```python
from build123d import *

# Parameters (mm, degrees)
EXTRUDE_1_OUTLINE_R   = 35
EXTRUDE_1_OUTLINE_R_2 = 1.55
EXTRUDE_1_OUTLINE_R_3 = 30.05
EXTRUDE_1_DEPTH       = 10
SKETCH_2_R            = 33.525
SKETCH_2_R_2          = 18.525
EXTRUDE_1_2_DEPTH     = 4
SKETCH_3_R            = 1.55
CUT_EXTRUDE_1_DEPTH   = 51.497524692
CUT_EXTRUDE_2_DEPTH   = 6
SKETCH_8_R            = 35
SKETCH_8_R_2          = 30.05
CUT_EXTRUDE_3_DEPTH   = 2
SKETCH_9_R            = 3
CUT_EXTRUDE_4_DEPTH   = 2
SKETCH_10_R           = 1.55
CUT_EXTRUDE_5_DEPTH   = 51.139804547
SKETCH_11_R           = 3
CUT_EXTRUDE_6_DEPTH   = 2


# Read off the part's stored shape, not the designer's step: 凸台-拉伸1
with BuildPart() as part:
    # Extrude 1 outline → Extrude 1 (new body)
    with BuildSketch(Plane.XY):
        Circle(EXTRUDE_1_OUTLINE_R)
        with Locations((0, -32.5)):
            Circle(EXTRUDE_1_OUTLINE_R_2, mode=Mode.SUBTRACT)
        with Locations((-32.5, 0)):
            Circle(EXTRUDE_1_OUTLINE_R_2, mode=Mode.SUBTRACT)
        Circle(EXTRUDE_1_OUTLINE_R_3, mode=Mode.SUBTRACT)
        with Locations((32.5, 0)):
            Circle(EXTRUDE_1_OUTLINE_R_2, mode=Mode.SUBTRACT)
        with Locations((0, 32.5)):
            Circle(EXTRUDE_1_OUTLINE_R_2, mode=Mode.SUBTRACT)
    extrude(amount=EXTRUDE_1_DEPTH)

    # 草图2 → Extrude 1 2 (add)
    with BuildSketch(Plane.XY.offset(10)):
        Circle(SKETCH_2_R)
        Circle(SKETCH_2_R_2, mode=Mode.SUBTRACT)
    extrude(amount=-EXTRUDE_1_2_DEPTH)

    # 草图3 → 切除-拉伸1 (cut, through all)
    with BuildSketch(Plane(origin=(0, 0, 0), x_dir=(-1, 0, 0), z_dir=(0, 0, -1))):
        with Locations(Location((32.5, 0, 0), (0, 0, 180))):
            Circle(SKETCH_3_R)
        with Locations(Location((0, -32.5, 0), (0, 0, 180))):
            Circle(SKETCH_3_R)
        with Locations(Location((-32.5, 0, 0), (0, 0, 180))):
            Circle(SKETCH_3_R)
        with Locations(Location((0, 32.5, 0), (0, 0, 180))):
            Circle(SKETCH_3_R)
    extrude(amount=-CUT_EXTRUDE_1_DEPTH, mode=Mode.SUBTRACT)

    # 草图7 → 切除-拉伸2 (cut)
    with BuildSketch(Plane(origin=(0, 0, 0), x_dir=(-1, 0, 0), z_dir=(0, 0, -1))):
        with BuildLine():
            Line((15.025, 26.024063384), (17.5, 30.310889132))
            ThreePointArc((17.5, 30.310889132), (24.748737342, 24.748737342), (30.310889132, 17.5))
            Line((30.310889132, 17.5), (26.024063384, 15.025))
            ThreePointArc((26.024063384, 15.025), (21.248558775, 21.248558775), (15.025, 26.024063384))
        make_face()
    extrude(amount=-CUT_EXTRUDE_2_DEPTH, mode=Mode.SUBTRACT)

    # 草图8 → 切除-拉伸3 (cut)
    with BuildSketch(Plane(origin=(0, 0, 0), x_dir=(-1, 0, 0), z_dir=(0, 0, -1))):
        with Locations(Location((0, 0, 0), (0, 0, 30))):
            Circle(SKETCH_8_R)
        Circle(SKETCH_8_R_2, mode=Mode.SUBTRACT)
    extrude(amount=-CUT_EXTRUDE_3_DEPTH, mode=Mode.SUBTRACT)

    # 草图9 → 切除-拉伸4 (cut)
    with BuildSketch(Plane.XY.offset(10)):
        with Locations((0, 32.5)):
            Circle(SKETCH_9_R)
        with Locations((32.5, 0)):
            Circle(SKETCH_9_R)
        with Locations((0, -32.5)):
            Circle(SKETCH_9_R)
        with Locations((-32.5, 0)):
            Circle(SKETCH_9_R)
    extrude(amount=-CUT_EXTRUDE_4_DEPTH, mode=Mode.SUBTRACT)

    # 草图10 → 切除-拉伸5 (cut, through all)
    with BuildSketch(Plane.XY.offset(10)):
        with Locations((22.980970389, 22.980970389)):
            Circle(SKETCH_10_R)
        with Locations((22.980970389, -22.980970389)):
            Circle(SKETCH_10_R)
        with Locations((-22.980970389, -22.980970389)):
            Circle(SKETCH_10_R)
        with Locations((-22.980970389, 22.980970389)):
            Circle(SKETCH_10_R)
    extrude(amount=-CUT_EXTRUDE_5_DEPTH, mode=Mode.SUBTRACT)

    # 草图11 → 切除-拉伸6 (cut)
    with BuildSketch(Plane.XY.offset(10)):
        with Locations((22.980970389, 22.980970389)):
            Circle(SKETCH_11_R)
        with Locations((22.980970389, -22.980970389)):
            Circle(SKETCH_11_R)
        with Locations((-22.980970389, -22.980970389)):
            Circle(SKETCH_11_R)
        with Locations((-22.980970389, 22.980970389)):
            Circle(SKETCH_11_R)
    extrude(amount=-CUT_EXTRUDE_6_DEPTH, mode=Mode.SUBTRACT)


solid = part.part
```
Design review of the part built by this model. Coordinates are the model's own, in mm. A direction names the side the tool comes from. Round coordinates to 2 decimals unless told otherwise and drop trailing zeros. Order: outer loops, then holes, each group sorted by start corner. A loop starts at its lowest first (then second) coordinate and runs counter-clockwise, first axis right, second up. Notation, with made-up numbers: M 27,28 L 63,28 A13 cw 63,46 Z; hole C 60.5,56.25 d1. An arc over 180 degrees is marked long. Put each result on its own line as item: value.
Q1. To check wall thickness, follow line 1 (X direction, y = 0, z = 3.25); line 2 (Y direction, x = 23, z = 4.5); line 3 (Y direction, x = 0, z = 8.5) (3 decimals). State the ranges of each line that lie inside material, in increasing order.
Reported:
line 1: -35 to -34.05, -30.95 to -30.05, 30.05 to 30.95, 34.05 to 35
line 2: -26.38 to -24.53, -21.43 to -19.34, 19.34 to 21.43, 24.53 to 26.38
line 3: -29.5 to -18.525, 18.525 to 29.5
Q2. Consider section A-A (y = -15.5). State the section outline as (x, z) points, and give its area (3 significant figures).
Reported:
outline: M -31.38,2 L -25.74,2 L -25.74,6 L -10.15,6 L -10.15,10 L -31.38,10 Z; M 10.15,6 L 25.74,6 L 25.74,2 L 31.38,2 L 31.38,10 L 10.15,10 Z
area: 215 mm²
Q3. Insertion check: pin 1 Ø5 at (x, y) = (0, -32.5) entering from +Z; pin 2 Ø5 at (x, y) = (-22.5, 22.5) entering from +Z; pin 3 Ø1 at (y, z) = (-26.5, 7.5) entering from -X; pin 4 Ø4 at (x, z) = (-27, 3) entering from +Y. Each pin has a flat end and moves straight along its axis. Give the tip position at first contact, or say it passes through.
Reported:
pin 1: z = 8
pin 2: z = 10
pin 3: x = -23.43
pin 4: y = 16.74
Q4. Consider section D-D (z = 3.25). State the section outline as (x, y) points (3 decimals).
Reported:
outline: M -30.311,17.5 A35 ccw long -17.5,30.311 L -15.025,26.024 A30.05 cw long -26.024,15.025 Z; hole C -32.5,0 d3.1; hole C -22.981,-22.981 d3.1; hole C 0,-32.5 d3.1; hole C 0,32.5 d3.1; hole C 22.981,-22.981 d3.1; hole C 22.981,22.981 d3.1; hole C 32.5,0 d3.1
Q5. Machinability: for faces 1 (the face through (20.37, -22.09, 3.97)), 2 (the face through (29.5, 0.1, 9)), 3 (the face through (21.84, -21.93, 5.04)), which of the approach directions +Z, -Z, +X, -X, +Y, -Y give a long, thin tool a straight path to every point of the face, cutting with its end or side? Answer none if there is none.
Reported:
face 1: -Z
face 2: +Z
face 3: +Z, -Z
Q6. Consider section B-B (x = 7.5). State the section outline as (y, z) points.
Reported:
outline: M -34.19,2 L -29.1,2 L -29.1,6 L -16.94,6 L -16.94,10 L -34.19,10 Z; M 16.94,6 L 29.1,6 L 29.1,2 L 34.19,2 L 34.19,10 L 16.94,10 Z
Q7. Draft analysis for pull direction X (two halves, no side actions). For faces 4 (the face through (-28.2, 16.28, 3.97)), 5 (the face through (-16.245, 28.137, 3.972)), state which applies: released by +X, released by -X, zero draft, split by the parting line, or undercut.
Reported:
face 4: undercut
face 5: released by -X
Q8. Consider section C-C (y = 0). State the section outline as (x, z) points (3 decimals).
Reported:
outline: M -35,2 L -34.05,2 L -34.05,8 L -35,8 Z; M -30.95,2 L -30.05,2 L -30.05,6 L -18.525,6 L -18.525,10 L -29.5,10 L -29.5,8 L -30.95,8 Z; M 18.525,6 L 30.05,6 L 30.05,2 L 30.95,2 L 30.95,8 L 29.5,8 L 29.5,10 L 18.525,10 Z; M 34.05,2 L 35,2 L 35,8 L 34.05,8 Z
